Check sheet for the drawn part. Datum: minimum x, y, z corner. Units: mm. A direction names the side the tool comes from. Give positions to 0.01 mm unless a question says otherwise; leave off trailing zeros. Order: outer loops, then holes, each group sorted by start corner. A loop starts at its lowest first (then second) coordinate and runs counter-clockwise, first axis right, second up. Notation, with made-up numbers: (-12, 75) - (11, 75) arc R19 cw to (11, 109) - close; hole circle Ø7 at (18, 83). An arc over 180 degrees is marked (long way). Answer as a JSON object with one key per item and string values. Group by question number.
(1) Section check B-B (x = 30). Record the boundary of the cut face in (y, z), then the cut area to 3 significant figures.
(2) Section check D-D (y = 2.5). Record the boundary of the cut face in (x, z).
(3) Depth check by flat-ended pin: pin 1 Ø2 at (x, y) = (11.5, 17.5) entering from -Z. Enter the tip coordinate at first touch or a pass-through.
(4) Section check A-A (y = 10). Record the boundary of the cut face in (x, z).
(5) Thickness scan on line 1 (Y direction, x = 10, z = 2.15); line 2 (X direction, y = 12.25, z = 0.8); line 3 (X direction, y = 8, z = 2.4). Record the ranges inside material, lowest first.
(6) Section check C-C (z = 0.9). Record the boundary of the cut face in (x, y), then the cut area to 3 significant figures.
(7) Mould release check, pull along X, two halves, no side actions. Record for the marked faces 1, 2 and 3: +X half, -X half, draft (parallel to the pull), parting line (faces both ways), or undercut.
(8) Access from +Z, -Z, +X, -X, +Y, -Y to the whole of each face (thin tool, end or side, straight path). Record for the marked faces 4 and 5.
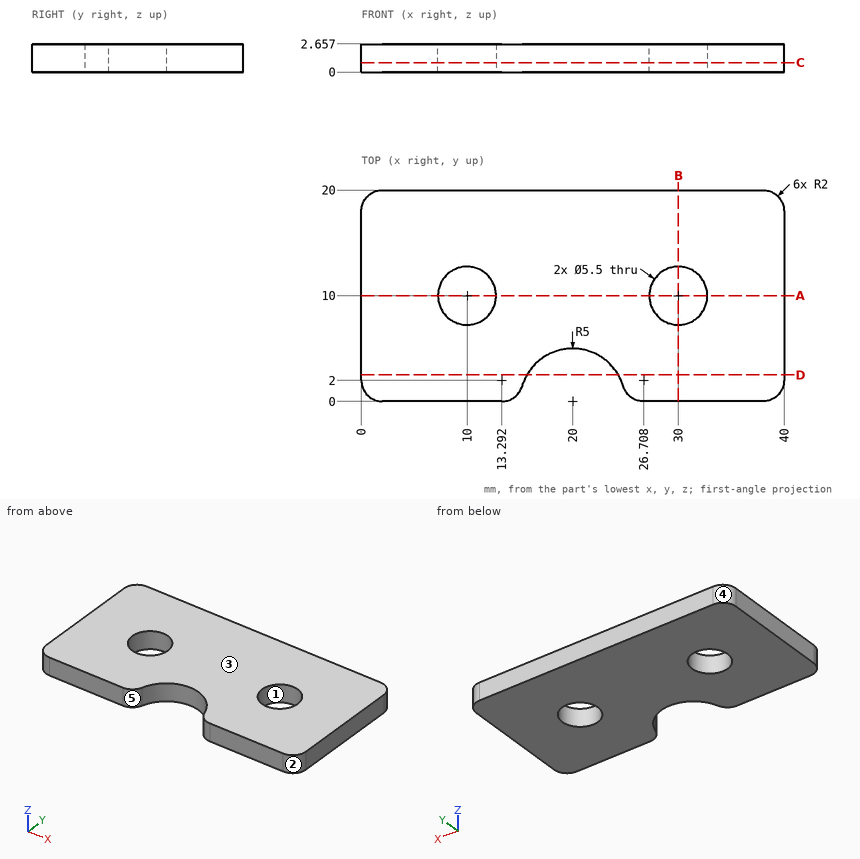
Solutions:
{
 "1": {"outline": "(0, 0) - (7.25, 0) - (7.25, 2.66) - (0, 2.66) - close; (12.75, 0) - (20, 0) - (20, 2.66) - (12.75, 2.66) - close", "area": "38.5 mm2"},
 "2": {"outline": "(0, 0) - (15.67, 0) - (15.67, 2.66) - (0, 2.66) - close; (24.33, 0) - (40, 0) - (40, 2.66) - (24.33, 2.66) - close"},
 "3": {"pin 1": "stops at z = 0"},
 "4": {"outline": "(0, 0) - (7.25, 0) - (7.25, 2.66) - (0, 2.66) - close; (12.75, 0) - (27.25, 0) - (27.25, 2.66) - (12.75, 2.66) - close; (32.75, 0) - (40, 0) - (40, 2.66) - (32.75, 2.66) - close"},
 "5": {"line 1": "y = 0 to 7.25, 12.75 to 20", "line 2": "x = 0 to 8.42, 11.58 to 28.42, 31.58 to 40", "line 3": "x = 0 to 8.11, 11.89 to 28.11, 31.89 to 40"},
 "6": {"outline": "(0, 2) arc R2 ccw to (2, 0) - (13.29, 0) arc R2 ccw to (15.21, 1.43) arc R5 cw to (24.79, 1.43) arc R2 ccw to (26.71, 0) - (38, 0) arc R2 ccw to (40, 2) - (40, 18) arc R2 ccw to (38, 20) - (2, 20) arc R2 ccw to (0, 18) - close; hole circle Ø5.5 at (10, 10); hole circle Ø5.5 at (30, 10)", "area": "709 mm2"},
 "7": {"face 1": "undercut", "face 2": "+X half", "face 3": "draft"},
 "8": {"face 4": "+Z, -Z, -X, +Y", "face 5": "+Z, -Z, -Y"}
}
